```python
from build123d import *

# Parameters (mm, degrees)
SKETCH2_W           = 80.5
SKETCH2_H           = 60
SKETCH2_R           = 1.8
BOSS_EXTRUDE1_DEPTH = 2.4
SKETCH2_3_W         = 4
SKETCH2_3_H         = 3
SKETCH2_3_H_2       = 4
SKETCH2_3_W_2       = 3
BOSS_EXTRUDE2_DEPTH = 12.5
SKETCH3_W           = 4
SKETCH3_H           = 7
SKETCH3_W_2         = 7
SKETCH3_H_2         = 4
BOSS_EXTRUDE3_DEPTH = 3


with BuildPart() as part:
    # Sketch2 → Boss-Extrude1 (new body)
    with BuildSketch(Plane(origin=(0, 0, 0), x_dir=(1, 0, 0), z_dir=(0, 1, 0))):
        Rectangle(SKETCH2_W, SKETCH2_H)
        with Locations(Location((-32.25, -22, 0), (0, 0, 270))):
            Circle(SKETCH2_R, mode=Mode.SUBTRACT)
        with Locations(Location((32.25, -22, 0), (0, 0, 270))):
            Circle(SKETCH2_R, mode=Mode.SUBTRACT)
        with Locations(Location((32.25, 22, 0), (0, 0, 270))):
            Circle(SKETCH2_R, mode=Mode.SUBTRACT)
        with Locations(Location((-32.25, 22, 0), (0, 0, 270))):
            Circle(SKETCH2_R, mode=Mode.SUBTRACT)
    extrude(amount=BOSS_EXTRUDE1_DEPTH)

    # Sketch2_3 → Boss-Extrude2 (add)
    with BuildSketch(Plane(origin=(0, 0, 0), x_dir=(1, 0, 0), z_dir=(0, 1, 0))):
        with Locations((0, -28.5)):
            Rectangle(SKETCH2_3_W, SKETCH2_3_H)
        with Locations((38.25, 0)):
            Rectangle(SKETCH2_3_W, SKETCH2_3_H_2)
        with Locations((0, 28.5)):
            Rectangle(SKETCH2_3_W, SKETCH2_3_H)
        with Locations((-38.75, 0)):
            Rectangle(SKETCH2_3_W_2, SKETCH2_3_H_2)
    extrude(amount=BOSS_EXTRUDE2_DEPTH)

    # Sketch3 → Boss-Extrude3 (add)
    with BuildSketch(Plane(origin=(0, 12.5, 0), x_dir=(1, 0, 0), z_dir=(0, 1, 0))):
        with Locations((0, 26.5)):
            Rectangle(SKETCH3_W, SKETCH3_H)
        with Locations((-36.75, 0)):
            Rectangle(SKETCH3_W_2, SKETCH3_H_2)
        with Locations((0, -26.5)):
            Rectangle(SKETCH3_W, SKETCH3_H)
        with Locations((36.75, 0)):
            Rectangle(SKETCH3_W_2, SKETCH3_H_2)
    extrude(amount=BOSS_EXTRUDE3_DEPTH)


solid = part.part
```
Geometry check sheet. Reference: the model listing, model coordinates, mm. A direction names the side the tool comes from. Coordinates: 2 decimals unless noted, no trailing zeros. Order: outer loops, then holes, each group sorted by start corner. A loop starts at its lowest first (then second) coordinate and runs counter-clockwise, first axis right, second up.
Item 1: Depth check by flat-ended pin: pin 1 (5.5 mm diameter, centred on y = 12, z = 25.5, fed in from -X); pin 2 (4 mm diameter, centred on x = 32.25, z = -22, fed in from +Y); pin 3 (5.5 mm diameter, centred on y = 9, z = -25.5, fed in from +X). Enter the tip coordinate at first touch or a pass-through.
Item 2: Mould release check, pull along X, two halves, no side actions. Record for faces 1 (the flat face through (40.25, 3, 0)), 2 (the flat face through (-40.25, 3, 0)), 3 (the flat face through (-35, 12.5, 0)): released by +X, released by -X, zero draft, split by the parting line, or undercut.
Item 3: Tool access check on faces 4 (the flat face through (2, 10, -28)), 5 (the flat face through (-33.25, 14, 0)), 6 (the flat face through (37, 10, -2)), 7 (the flat face through (0, 7, -27)), 8 (the flat face through (37, 10, 2)). Record the directions out of +Z, -Z, +X, -X, +Y, -Y that give a thin tool (end or side, any length) a straight path to the whole face; none if there is none.
Item 4: Section check D-D (y = 13.5). Enter the section's corners in (x, z).
Item 5: Section check C-C (z = -22). Enter the section's corners in (x, y).
Item 6: Section check B-B (y = 6.5). Enter the section's corners in (x, z), plus the area to 3 significant figures.
Item 7: Section check A-A (x = -32.25). Enter the section's corners in (y, z).
Item 8: Scan lines: line 1 along X through (y, z) = (0.85, 22); line 2 along Y through (x, z) = (-14.5, 2); line 3 along X through (y, z) = (14.75, -25.5). Record each from-to range of solid material in increasing order.
Check sheet entries:
1. pin 1: stops at x = -2
1. pin 2: stops at y = 2.4
1. pin 3: stops at x = 2
2. face 1: released by +X
2. face 2: released by -X
2. face 3: undercut
3. face 4: +Z, -Z, +X, +Y
3. face 5: +Z, -Z, +Y
3. face 6: -Z, +X, -X, +Y
3. face 7: +X, -X
3. face 8: +Z, +X, -X, +Y
4. outline: (-40.25, -2) - (-33.25, -2) - (-33.25, 2) - (-40.25, 2) - close; (-2, -30) - (2, -30) - (2, -23) - (-2, -23) - close; (-2, 23) - (2, 23) - (2, 30) - (-2, 30) - close; (33.25, -2) - (40.25, -2) - (40.25, 2) - (33.25, 2) - close
5. outline: (-40.25, 0) - (-34.05, 0) - (-34.05, 2.4) - (-40.25, 2.4) - close; (-30.45, 0) - (30.45, 0) - (30.45, 2.4) - (-30.45, 2.4) - close; (34.05, 0) - (40.25, 0) - (40.25, 2.4) - (34.05, 2.4) - close
6. outline: (-40.25, -2) - (-37.25, -2) - (-37.25, 2) - (-40.25, 2) - close; (-2, -30) - (2, -30) - (2, -27) - (-2, -27) - close; (-2, 27) - (2, 27) - (2, 30) - (-2, 30) - close; (36.25, -2) - (40.25, -2) - (40.25, 2) - (36.25, 2) - close
6. area: 52.0 mm2
7. outline: (0, -30) - (2.4, -30) - (2.4, -23.8) - (0, -23.8) - close; (0, -20.2) - (2.4, -20.2) - (2.4, 20.2) - (0, 20.2) - close; (0, 23.8) - (2.4, 23.8) - (2.4, 30) - (0, 30) - close
8. line 1: x = -40.25 to -34.05, -30.45 to 30.45, 34.05 to 40.25
8. line 2: y = 0 to 2.4
8. line 3: x = -2 to 2
